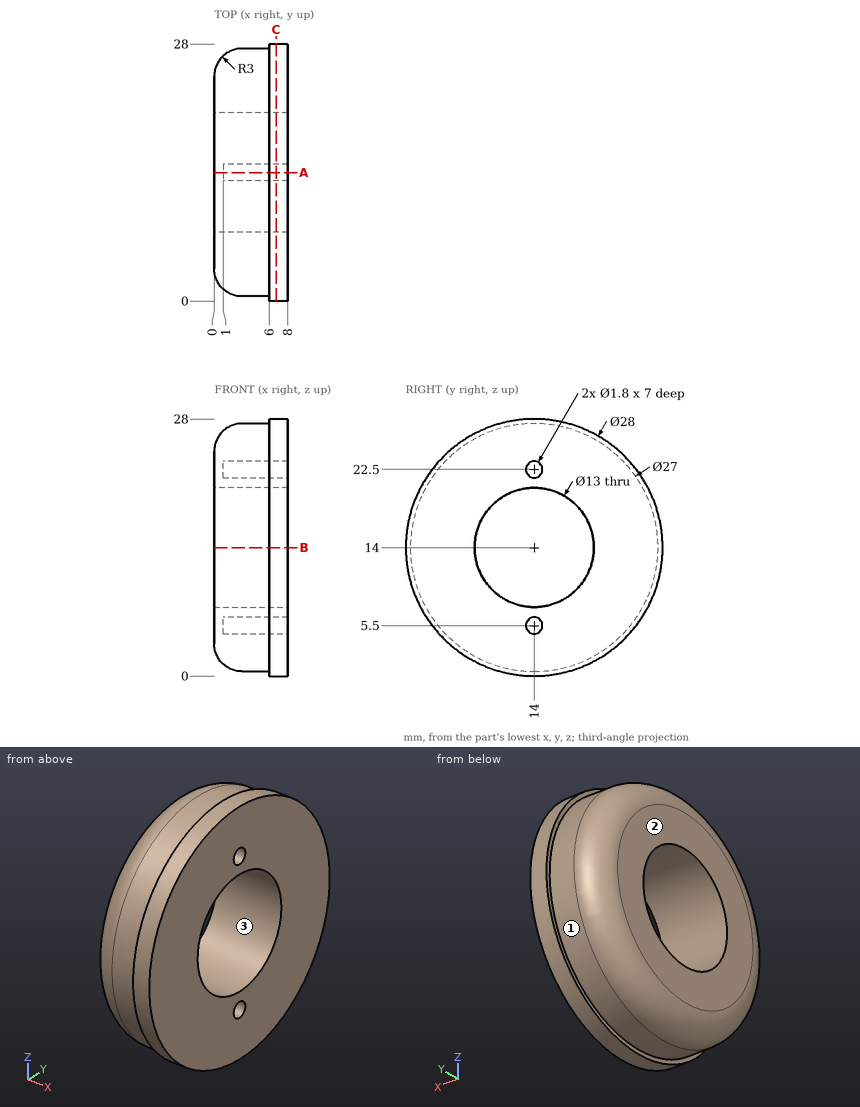
Answer from the drawing. Dimensions are ordinates in mm from the lowest x, y and z of the part. Coordinates: 2 decimals unless noted, no trailing zeros. Write each loop counter-clockwise with the first axis right and the second up, starting at its lowest first coordinate (ties: lowest second). Pieces come first, ordered by that corner, then holes. Notation, with made-up numbers: (-20, 50) - (26, 50) arc R27 cw to (26, 82) - close; hole circle Ø1 at (8, 13.5). An arc over 180 degrees is marked (long way). Return JSON: item names as keys, results as strings. Group by question number.
Q1. The part is cut by section C-C on x = 6.75. Write down the section's boundary in (y, z), and give its area (3 significant figures).
Q2. Flat-ended cylindrical pins translate along their axes: pin 1 Ø1.6 at (y, z) = (14, 22.5) entering from +X; pin 2 Ø1 at (x, z) = (4.5, 5.5) entering from -Y; pin 3 Ø1.5 at (x, y) = (5.5, 3) entering from +Z. Find the tip coordinate at first contact, or state that the pin passes through.
Q3. Find the intervals of material crossed by line 1 along Y through (x, z) = (6.5, 14); line 2 along Y through (x, z) = (5, 14); line 3 along Z through (x, y) = (3.5, 14.75), in increasing order. Write a range as [from, to].
Q4. The part is cut by section A-A on y = 14. Write down the section's boundary in (x, z), and give its area (3 significant figures).
Q5. The part is cut by section B-B on z = 14. Write down the section's boundary in (x, y).
Q6. For a pull along Z with two mould halves and no side action, classify the marked faces 1, 2 and 3 as +Z half, -Z half, draft (parallel to the pull), parting line (faces both ways), or undercut.
Evaluation:
{
 "1": {"outline": "circle Ø28 at (14, 14); hole circle Ø13 at (14, 14); hole circle Ø1.8 at (14, 5.5); hole circle Ø1.8 at (14, 22.5)", "area": "478 mm2"},
 "2": {"pin 1": "stops at x = 1", "pin 2": "stops at y = 3.13", "pin 3": "stops at z = 23.33"},
 "3": {"line 1": "y = [0, 7.5], [20.5, 28]", "line 2": "y = [0.5, 7.5], [20.5, 27.5]", "line 3": "z = [0.52, 5], [6, 7.54], [20.46, 22], [23, 27.48]"},
 "4": {"outline": "(0, 3.5) arc R3 ccw to (3, 0.5) - (6, 0.5) - (6, 0) - (8, 0) - (8, 4.6) - (1, 4.6) - (1, 6.4) - (8, 6.4) - (8, 7.5) - (0, 7.5) - close; (0, 20.5) - (8, 20.5) - (8, 21.6) - (1, 21.6) - (1, 23.4) - (8, 23.4) - (8, 28) - (6, 28) - (6, 27.5) - (3, 27.5) arc R3 ccw to (0, 24.5) - close", "area": "84.9 mm2"},
 "5": {"outline": "(0, 3.5) arc R3 ccw to (3, 0.5) - (6, 0.5) - (6, 0) - (8, 0) - (8, 7.5) - (0, 7.5) - close; (0, 20.5) - (8, 20.5) - (8, 28) - (6, 28) - (6, 27.5) - (3, 27.5) arc R3 ccw to (0, 24.5) - close"},
 "6": {"face 1": "parting line", "face 2": "draft", "face 3": "undercut"}
}
